Source: CAD feature listing. Evaluate the final solid. Frame: model axes, mm. A direction names the side the tool comes from. Coordinates: 2 decimals unless noted, no trailing zeros. Loops run counter-clockwise (first coordinate to the right, second up) from the corner with the lowest first, then second, coordinate; pieces in that order, holes last.
from build123d import *

# Parameters (mm, degrees)
EXTRUDE_1_DEPTH          = 2
CUT_EXTRUDE_1_DEPTH      = 106.5
CUT_EXTRUDE_1_DEPTH_BACK = 62.743635726


with BuildPart() as part:
    # Эскиз1 → Бобышка-Вытянуть1 (new body)
    with BuildSketch(Plane(origin=(0, 0, 0), x_dir=(1, 0, 0), z_dir=(0, 1, 0))):
        with BuildLine():
            Line((-56.923759365, -23.831956958), (16.382902061, -23.831956958))
            Line((16.382902061, -23.831956958), (-0.836945892, -15.802209985))
            Line((-0.836945892, -15.802209985), (-17.271974735, 0.632818857))
            Line((-17.271974735, 0.632818857), (-55.146365247, 0.632818857))
            ThreePointArc((-55.146365247, 0.632818857), (-50.679018006, -7.808361393), (-51.74094673, -17.29956905))
            ThreePointArc((-51.74094673, -17.29956905), (-53.905020217, -20.904809923), (-56.923759365, -23.831956958))
        make_face()
        Polygon((-19.117097939, -17.29956905), (-49.391279562, -17.29956905), (-49.391279562, -8.89956905), (-27.396659044, -8.89956905), (-19.117097939, -8.89956905), align=None, mode=Mode.SUBTRACT)
    extrude(amount=EXTRUDE_1_DEPTH)

    # Эскиз2 → Вырез-Вытянуть1 (cut, two sides: drawn at the far end of the back side and taken through both)
    with BuildSketch(Plane(origin=(0, 2, 0), x_dir=(1, 0, 0), z_dir=(0, 1, 0)).offset(-CUT_EXTRUDE_1_DEPTH_BACK)):
        Polygon((16.382902061, -23.831956958), (15.960145161, -23.634822178), (16.059019052, -23.90647596), align=None)
    extrude(amount=CUT_EXTRUDE_1_DEPTH + CUT_EXTRUDE_1_DEPTH_BACK, mode=Mode.SUBTRACT)


solid = part.part
Q1. Section B-B, the plane y = 0.85. Return the cut outline in (x, z).
Q2. Section C-C, the plane z = 12.75. Return the cut outline in (x, y), plus the area to 3 significant figures.
Q3. Draft query along X for faces 3 (the flat face through (-34, 1, 17.3)), 4 (the flat face through (-8.94, 0.99, 7.7)), 5 (the flat face through (-21, 1, 23.832)). Return one class per face: +X half, -X half, draft (parallel to the pull), parting line (faces both ways), or undercut.
Q4. Section A-A, the plane x = -48. Return the cut outline in (y, z), plus the area to 3 significant figures.
Q5. Section D-D, the plane x = -15. Return the cut outline in (y, z).
Q6. Contact query for a flat-ended pin moving along its axis: pin 1 Ø1 at (y, z) = (1.5, 12) entering from -X. Output: stop coordinate, or through.
Q7. Access query for faces 1 (the flat face through (-21, 0, 8.7)), 2 (the flat face through (-34, 1, 8.9)). Directions: +Z, -Z, +X, -X, +Y, -Y. A direction counts if a zero-diameter tool reaches every point of the face in a straight line with its end or side. Return the directions, or none.
Q8. Line query: line 1 along Z through (x, y) = (-35, 1.5); line 2 along X through (y, z) = (1.35, 16.75); line 3 along X through (y, z) = (0.5, 13.5). Output: solid intervals per line, ascending.
Derived:
1. outline: (-56.92, 23.83) arc R16.21 cw to (-55.15, -0.63) - (-17.27, -0.63) - (-0.84, 15.8) - (15.96, 23.63) - (16.03, 23.83) - close; hole (-49.39, 8.9) - (-19.12, 8.9) - (-19.12, 17.3) - (-49.39, 17.3) - close
2. outline: (-50.51, 0) - (-49.39, 0) - (-49.39, 2) - (-50.51, 2) - close; (-19.12, 0) - (-3.89, 0) - (-3.89, 2) - (-19.12, 2) - close
2. area: 32.7 mm2
3. face 3: undercut
3. face 4: +X half
3. face 5: draft
4. outline: (0, -0.63) - (2, -0.63) - (2, 8.9) - (0, 8.9) - close; (0, 17.3) - (2, 17.3) - (2, 23.83) - (0, 23.83) - close
4. area: 32.1 mm2
5. outline: (0, 1.64) - (2, 1.64) - (2, 23.83) - (0, 23.83) - close
6. pin 1: stops at x = -50.48
7. face 1: +Z, -Z, +X, -X, -Y
7. face 2: +Y, -Y
8. line 1: z = -0.63 to 8.9, 17.3 to 23.83
8. line 2: x = -51.51 to -49.39, -19.12 to 1.2
8. line 3: x = -50.62 to -49.39, -19.12 to -3.14
